The model under review builds one solid part; all positions refer to its coordinate system, in mm. Face numbers are marked on the shaded views. Give positions to 0.01 mm unless a question says otherwise; leave off trailing zeros. Loops run counter-clockwise (first coordinate to the right, second up) from the corner with the lowest first, then second, coordinate; pieces in that order, holes last. Notation, with made-up numbers: M -25,24.25 L 12,24.25 A17 cw 12,55.25 Z; hole C 33.5,-9 d11. An arc over 180 degrees is marked long. Put each result on its own line as item: value. Start each with the question number.
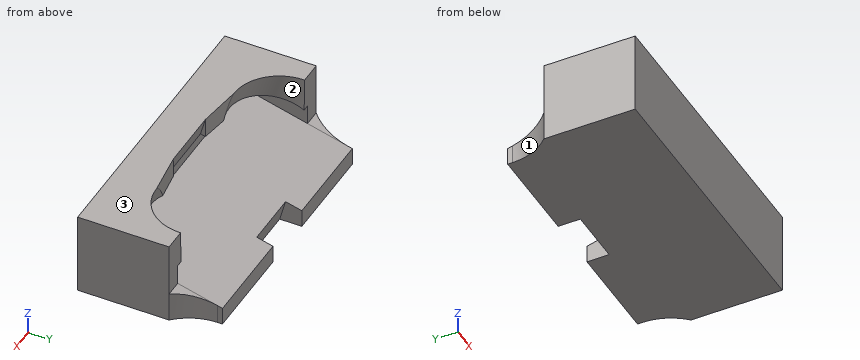
from build123d import *

# Parameters (mm, degrees)
SKETCH1_W           = 45
SKETCH1_H           = 15
BOSS_EXTRUDE1_DEPTH = 5
BOSS_EXTRUDE2_DEPTH = 45
SKETCH5_R           = 8
CUT_EXTRUDE1_DEPTH  = 10
CUT_EXTRUDE2_REACH  = 39.075
SKETCH6_W           = 45
SKETCH6_H           = 8
SKETCH7_W           = 11
SKETCH7_H           = 10.717790556
CUT_EXTRUDE4_DEPTH  = 6.5
CUT_EXTRUDE5_REACH  = 39.075
SKETCH10_W          = 15
SKETCH10_H          = 16.318516526
BOSS_EXTRUDE3_DEPTH = 3
SKETCH11_W          = 15
SKETCH11_H          = 16.318516526
BOSS_EXTRUDE4_DEPTH = 3
SKETCH12_W          = 10
SKETCH12_H          = 7.679226714
CUT_EXTRUDE6_DEPTH  = 6
FILLET1_R           = 10


with BuildPart() as part:
    # Sketch1 → Boss-Extrude1 (new body)
    with BuildSketch(Plane(origin=(0, 0, 0), x_dir=(1, 0, 0), z_dir=(0, 1, 0))):
        with Locations((1.125, 2.045454545)):
            Rectangle(SKETCH1_W, SKETCH1_H)
    extrude(amount=BOSS_EXTRUDE1_DEPTH)

    # Sketch2 → Boss-Extrude2 (add)
    with BuildSketch(Plane(origin=(23.625, 0, 0), x_dir=(0, 0, -1), z_dir=(1, 0, 0))):
        Polygon((-2.454545455, 5), (2.721835448, 24.318516526), (-5.454545455, 24.318516526), (-5.454545455, 5), align=None)
        Polygon((1.168921177, 5), (6.345302079, 24.318516526), (9.545454545, 24.318516526), (9.545454545, 5), align=None)
    extrude(amount=-BOSS_EXTRUDE2_DEPTH)

    # Sketch5 → Cut-Extrude1 (cut)
    with BuildSketch(Plane(origin=(0, 0.948572854, 3.540122086), x_dir=(-1, 0, 0), z_dir=(0, -0.2588190451025247, -0.9659258262890673))):
        with Locations(Location((12.375, 14.194346021, 0), (0, 0, 90))):
            Circle(SKETCH5_R)
        with Locations(Location((-14.625, 14.194346021, 0), (0, 0, 90))):
            Circle(SKETCH5_R)
    extrude(amount=-CUT_EXTRUDE1_DEPTH, mode=Mode.SUBTRACT)

    # Cut-Extrude2: up to this plane
    cut_extrude2_end = Plane(origin=(-21.375, 5, 2.454545455), z_dir=(0, -0.2588190451025246, -0.9659258262890673))
    # Sketch6 → Cut-Extrude2 (cut, up to the surface)
    with BuildSketch(Plane.XY.offset(5.454545455), mode=Mode.PRIVATE) as cut_extrude2_sk1:
        with Locations((1.125, 20.318516526)):
            Rectangle(SKETCH6_W, SKETCH6_H)
    cut_extrude2_tool1 = split(extrude(cut_extrude2_sk1.sketch, amount=-CUT_EXTRUDE2_REACH, mode=Mode.PRIVATE), bisect_by=cut_extrude2_end, keep=Keep.BOTH, mode=Mode.PRIVATE)
    add(cut_extrude2_tool1.solids().sort_by_distance((1.125, 20.318517, 5.454545))[0], mode=Mode.SUBTRACT)

    # Sketch7 → Cut-Extrude4 (cut)
    with BuildSketch(Plane(origin=(0, 0.948572854, 3.540122086), x_dir=(-1, 0, 0), z_dir=(0, -0.2588190451025247, -0.9659258262890673))):
        with Locations((-1.125, 10.553241299)):
            Rectangle(SKETCH7_W, SKETCH7_H)
    extrude(amount=-CUT_EXTRUDE4_DEPTH, mode=Mode.SUBTRACT)


with BuildPart() as cut_extrude4_piece_1:
    # of the separate pieces the step leaves, piece 1, a body of its own (cut_extrude4_pieces)
    add(part.part.solids().sort_by_distance((-21.375, 0, -9.545454545))[0])


with BuildPart() as cut_extrude4_piece_2:
    # of the separate pieces the step leaves, piece 2, a body of its own (cut_extrude4_pieces)
    add(part.part.solids().sort_by_distance((-4.375, 16.318516526, -0.578241908))[0])


with BuildPart() as cut_extrude4_piece_3:
    # of the separate pieces the step leaves, piece 3, a body of its own (cut_extrude4_pieces)
    add(part.part.solids().sort_by_distance((6.811601533, 16.318516526, -0.578241908))[0])


with BuildPart() as cut_extrude5_tool:
    # Cut-Extrude5: up to this plane
    cut_extrude5_end = Plane(origin=(-21.375, 5, 2.454545455), z_dir=(0, -0.2588190451025246, -0.9659258262890673))
    # Sketch9 → Cut-Extrude5 (new, up to the surface)
    with BuildSketch(Plane.XY.offset(5.454545455), mode=Mode.PRIVATE) as cut_extrude5_sk1:
        Polygon((-12.375, 7.874399938), (-4.375, 6.839123758), (6.625, 6.839123758), (14.625, 7.874399938), (14.625, 17.142741254), (-12.375, 17.142741254), align=None)
    cut_extrude5_tool1 = split(extrude(cut_extrude5_sk1.sketch, amount=-CUT_EXTRUDE5_REACH, mode=Mode.PRIVATE), bisect_by=cut_extrude5_end, keep=Keep.BOTH, mode=Mode.PRIVATE)
    add(cut_extrude5_tool1.solids().sort_by_distance((1.125, 12.138424, 5.454545))[0])


with BuildPart() as cut_extrude4_piece_1_1:
    add(cut_extrude4_piece_1.part)

    # Cut-Extrude5: cut by cut_extrude5_tool
    add(cut_extrude5_tool.part, mode=Mode.SUBTRACT)

    # Sketch10 → Boss-Extrude3 (add)
    with BuildSketch(Plane.ZY.offset(21.375)):
        with Locations((-2.045454545, 8.159258263)):
            Rectangle(SKETCH10_W, SKETCH10_H)
    extrude(amount=BOSS_EXTRUDE3_DEPTH)

    # Sketch11 → Boss-Extrude4 (add)
    with BuildSketch(Plane(origin=(23.625, 0, 0), x_dir=(0, 0, -1), z_dir=(1, 0, 0))):
        with Locations((2.045454545, 8.159258263)):
            Rectangle(SKETCH11_W, SKETCH11_H)
    extrude(amount=BOSS_EXTRUDE4_DEPTH)

    # Sketch12 → Cut-Extrude6 (cut)
    with BuildSketch(Plane(origin=(0, 0.042706196, 0.159381694), x_dir=(1, 0, 0), z_dir=(0, 0.2588190451025247, 0.9659258262890673))):
        with Locations((1.125, 25.971781551)):
            Rectangle(SKETCH12_W, SKETCH12_H)
    extrude(amount=-CUT_EXTRUDE6_DEPTH, mode=Mode.SUBTRACT)

    # Fillet1
    # the kernel refuses this fillet: 10 mm, written as the material it adds along each edge
    with BuildSketch(Plane(origin=(-21.375, 16.318516526, 13.651862532), x_dir=(-1, 0, 0), z_dir=(0, 0, -1))) as fillet1_piece_1_section:
        with BuildLine():
            CenterArc((10, 7.141428429), FILLET1_R, 180, 45.572995999)
            Line((0, 7.141428429), (0, 0))
            Line((0, 0), (3, 0))
        make_face()
    fillet1_piece_1 = extrude(amount=23.197317077, mode=Mode.PRIVATE)
    fillet1_piece_1 = split(fillet1_piece_1, bisect_by=Plane(origin=(-22.137016454, 20.028758468, -5.195864872), z_dir=(0, -0.2588190451025247, -0.9659258262890673)), keep=Keep.TOP, mode=Mode.PRIVATE)
    add(fillet1_piece_1)
    with BuildSketch(Plane(origin=(23.625, 16.318516526, 13.651862532), x_dir=(1, 0, 0), z_dir=(0, 0, -1))) as fillet1_piece_2_section:
        with BuildLine():
            CenterArc((10, -7.141428429), FILLET1_R, 134.427004001, 45.572995999)
            Line((0, -7.141428429), (0, 0))
            Line((0, 0), (3, 0))
        make_face()
    fillet1_piece_2 = extrude(amount=23.197317077, mode=Mode.PRIVATE)
    fillet1_piece_2 = split(fillet1_piece_2, bisect_by=Plane(origin=(24.387016454, 20.028758468, -5.195864872), z_dir=(0, -0.2588190451025247, -0.9659258262890673)), keep=Keep.TOP, mode=Mode.PRIVATE)
    add(fillet1_piece_2)


with BuildPart() as cut_extrude4_piece_2_1:
    add(cut_extrude4_piece_2.part)

    # Cut-Extrude5: cut by cut_extrude5_tool
    add(cut_extrude5_tool.part, mode=Mode.SUBTRACT)


with BuildPart() as cut_extrude4_piece_3_1:
    add(cut_extrude4_piece_3.part)

    # Cut-Extrude5: cut by cut_extrude5_tool
    add(cut_extrude5_tool.part, mode=Mode.SUBTRACT)


solid = cut_extrude4_piece_1_1.part
(1) We need section C-C, the plane y = 19. Write out the cut boundary in (x, z) (3 decimals), plus the area to 3 significant figures.
(2) We need section A-A, the plane x = 18. Write out the cut boundary in (y, z).
(3) We need section D-D, the plane x = -11. Write out the cut boundary in (y, z), plus the area to 3 significant figures.
(4) We need section B-B, the plane z = -8.5. Write out the cut boundary in (x, y) (3 decimals).
(5) To check wall thickness, follow L1, parallel to X at y = 11.75, z = -2.75 (3 decimals); L2, parallel to Y at x = -3, z = 0.5; L3, parallel to Z at x = 0, y = 5.5. State the ranges of each line that lie inside material, in increasing order. Write a range as [from, to].
(6) Draft analysis for pull direction X (two halves, no side actions). For the marked faces 1, 2 and 3, state which applies: +X half, -X half, draft (parallel to the pull), parting line (faces both ways), or undercut.
(7) Insertion check: pin 1 (3 mm diameter, centred on x = -4.5, z = 4, fed in from +Y); pin 2 (0.7 mm diameter, centred on y = 24, z = -8.5, fed in from -X) (3 decimals); pin 3 (4 mm diameter, centred on y = 21.5, z = -2, fed in from +X); pin 4 (0.9 mm diameter, centred on y = 24, z = -8.5, fed in from +X) (3 decimals). Each pin has a flat end and moves straight along its axis. Give the tip position at first contact, or say it passes through.
Check sheet entries:
1. outline: M -22.425,-9.545 L 24.675,-9.545 L 24.675,-4.92 L -22.425,-4.92 Z
1. area: 218 mm²
2. outline: M 0,-9.55 L 24.32,-9.55 L 24.32,-6.35 L 5,-1.17 L 5,2.45 L 7.65,1.74 L 8.65,5.45 L 0,5.45 Z
3. outline: M 0,-9.55 L 24.32,-9.55 L 24.32,-6.35 L 5,-1.17 L 5,2.45 L 7.05,1.91 L 7.7,4.33 L 7.7,5.45 L 0,5.45 Z
3. area: 195 mm²
4. outline: M -24.375,0 L 26.625,0 L 26.625,16.319 A10 cw 23.625,23.46 L 23.625,24.319 L 6.125,24.319 L 6.125,20.635 L -3.875,20.635 L -3.875,24.319 L -21.375,24.319 L -21.375,23.46 A10 cw -24.375,16.319 Z
5. L1: x = [-24.375, -21.375], [23.625, 26.625]
5. L2: y = [0, 5]
5. L3: z = [-9.55, -1.3], [2.32, 5.45]
6. face 1: -X half
6. face 2: undercut
6. face 3: draft
7. pin 1: stops at y = 7.05
7. pin 2: stops at x = -21.375
7. pin 3: passes through
7. pin 4: stops at x = 23.625
